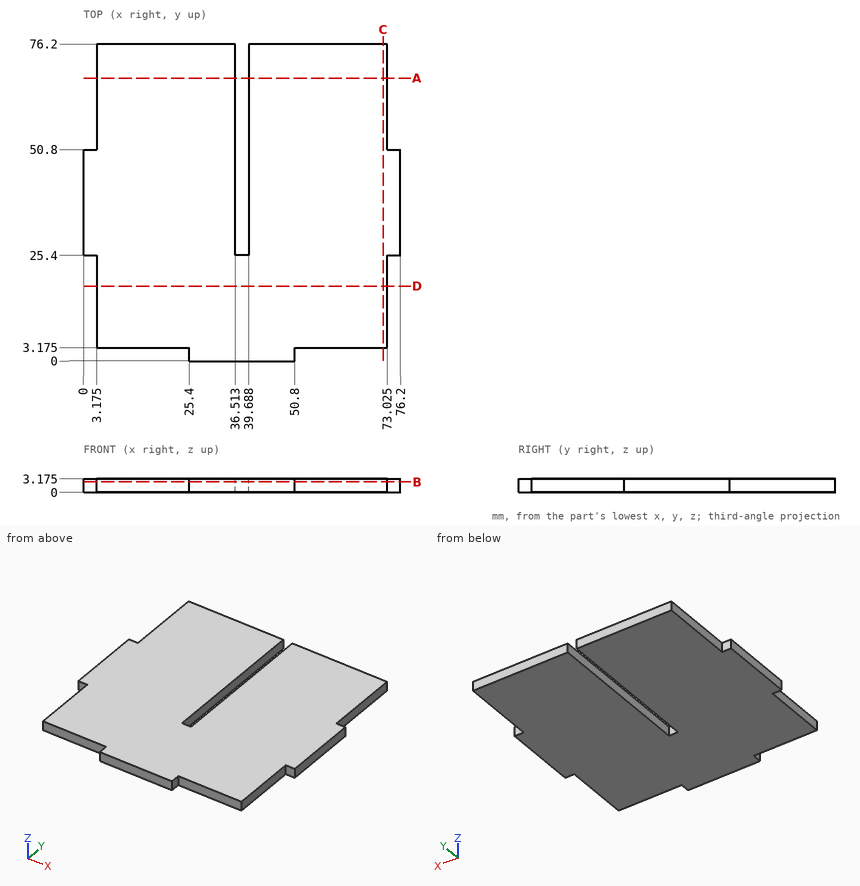
Design review of the part shown in the three views and the two pictorial views. Dimensions are in mm from the part's minimum x, y and z. Round coordinates to 2 decimals unless told otherwise and drop trailing zeros. Write each loop counter-clockwise with the first axis right and the second up, starting at its lowest first coordinate (ties: lowest second). Pieces come first, ordered by that corner, then holes. Notation, with made-up numbers: M 75.25,-6.75 L 98.25,-6.75 A24 ccw 98.25,7.25 Z; hole C 42,-34 d4. An arc over 180 degrees is marked long. Use a Markdown table: item, result. Add a question column.
Q1. We need section D-D, the plane y = 18. State the section outline as (x, z) points (1 decimal), plus the area to 3 significant figures.
Q2. To check wall thickness, follow line 1 (X direction, y = 35, z = 2.2); line 2 (X direction, y = 64, z = 2.9) (1 decimal); line 3 (Y direction, x = 70, z = 0.3) (1 decimal). State the ranges of each line that lie inside material, in increasing order.
Q3. We need section A-A, the plane y = 68. State the section outline as (x, z) points (1 decimal), plus the area to 3 significant figures.
Q4. Insertion check: pin 1 (1.6 mm diameter, centred on x = 66.5, z = 2.5, fed in from -Y) (1 decimal); pin 2 (1.6 mm diameter, centred on x = 1, z = 1, fed in from -Y); pin 3 (1 mm diameter, centred on y = 18, z = 1.5, fed in from +X) (1 decimal). Each pin has a flat end and moves straight along its axis. Give the tip position at first contact, or say it passes through.
Q5. We need section C-C, the plane x = 72. State the section outline as (y, z) points (1 decimal), plus the area to 3 significant figures.
Q6. We need section B-B, the plane z = 2.5. State the section outline as (x, y) points (1 decimal).
Findings below:
| question | item | result |
|---|---|---|
| 1 | outline | M 3.2,0 L 73,0 L 73,3.2 L 3.2,3.2 Z |
| 1 | area | 222 mm² |
| 2 | line 1 | x = 0 to 36.51, 39.69 to 76.2 |
| 2 | line 2 | x = 3.2 to 36.5, 39.7 to 73 |
| 2 | line 3 | y = 3.2 to 76.2 |
| 3 | outline | M 3.2,0 L 36.5,0 L 36.5,3.2 L 3.2,3.2 Z; M 39.7,0 L 73,0 L 73,3.2 L 39.7,3.2 Z |
| 3 | area | 212 mm² |
| 4 | pin 1 | stops at y = 3.2 |
| 4 | pin 2 | stops at y = 25.4 |
| 4 | pin 3 | stops at x = 73 |
| 5 | outline | M 3.2,0 L 76.2,0 L 76.2,3.2 L 3.2,3.2 Z |
| 5 | area | 232 mm² |
| 6 | outline | M 0,25.4 L 3.2,25.4 L 3.2,3.2 L 25.4,3.2 L 25.4,0 L 50.8,0 L 50.8,3.2 L 73,3.2 L 73,25.4 L 76.2,25.4 L 76.2,50.8 L 73,50.8 L 73,76.2 L 39.7,76.2 L 39.7,25.4 L 36.5,25.4 L 36.5,76.2 L 3.2,76.2 L 3.2,50.8 L 0,50.8 Z |
